Could you check a few things on this drawing? It's one solid part, dimensions in mm from its lowest x, y, z. A direction names the side the tool comes from. Round coordinates to 2 decimals unless told otherwise and drop trailing zeros. Order: outer loops, then holes, each group sorted by start corner. A loop starts at its lowest first (then second) coordinate and runs counter-clockwise, first axis right, second up.
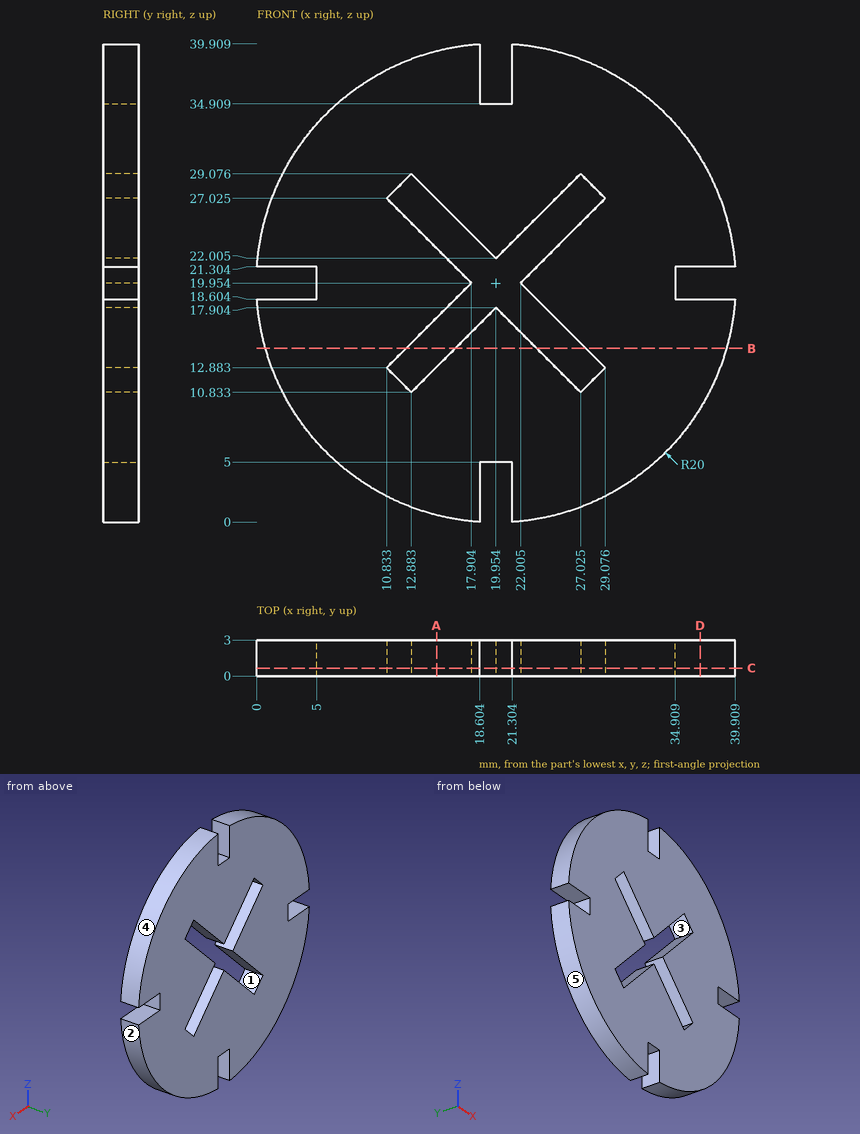
(1) I want a section at A-A, the plane x = 15. List the corners of the cut face in (y, z) for me.
(2) I'm going to push flat-ended pins straight in: pin 1 Ø1.4 at (x, y) = (19.5, 1) entering from -Z; pin 2 Ø0.9 at (y, z) = (1, 37.5) entering from -X (1 decimal); pin 3 Ø1.5 at (x, y) = (1.5, 1) entering from +Z (1 decimal). Where does each tip first touch, or does it pass through?
(3) I want a section at B-B, the plane z = 14.5. List the corners of the cut face in (x, y) for me.
(4) I want a section at D-D, the plane x = 37. List the corners of the cut face in (y, z) for me (1 decimal).
(5) If we mould it in two halves opening along X, with no side actions, what happens to the marked faces 3, 4 and 5? For each: pulls with the +X half, pulls with the -X half, needs draft (parallel to the pull), parting line crosses it, or undercut.
(6) Please list where these lines run through material, in increasing order: probe 1 along X at (y, z) = (1.6, 24); probe 2 along Z at (x, y) = (19, 1.5); probe 3 along Z at (x, y) = (2.5, 2.8) (1 decimal).
(7) On a 3-axis mill with a long thin cutter (end or side, diameter ignored), from which of +Z, -Z, +X, -X, +Y, -Y can I reach the whole of each face in a straight line? I mean the marked faces 1 and 2. Say none if no direction works.
(8) I want a section at C-C, the plane y = 0.65. List the corners of the cut face in (x, z) for me (1 decimal), plus the area to 3 significant figures.
Ans:
1. outline: (0, 0.58) - (3, 0.58) - (3, 12.95) - (0, 12.95) - close; (0, 17.05) - (3, 17.05) - (3, 22.86) - (0, 22.86) - close; (0, 26.96) - (3, 26.96) - (3, 39.33) - (0, 39.33) - close
2. pin 1: stops at z = 5
2. pin 2: stops at x = 9.6
2. pin 3: stops at z = 29.3
3. outline: (0.71, 0) - (12.45, 0) - (12.45, 3) - (0.71, 3) - close; (16.55, 0) - (23.36, 0) - (23.36, 3) - (16.55, 3) - close; (27.46, 0) - (39.2, 0) - (39.2, 3) - (27.46, 3) - close
4. outline: (0, 9.5) - (3, 9.5) - (3, 18.6) - (0, 18.6) - close; (0, 21.3) - (3, 21.3) - (3, 30.4) - (0, 30.4) - close
5. face 3: undercut
5. face 4: pulls with the +X half
5. face 5: pulls with the -X half
6. probe 1: x = 0.37 to 13.86, 17.96 to 21.95, 26.05 to 39.54
6. probe 2: z = 5 to 16.95, 22.96 to 34.91
6. probe 3: z = 10.2 to 18.6, 21.3 to 29.7
7. face 1: +Y, -Y
7. face 2: -Z, +X, +Y, -Y
8. outline: (0, 18.6) arc R20 ccw to (18.6, 0) - (18.6, 5) - (21.3, 5) - (21.3, 0) arc R20 ccw to (39.9, 18.6) - (34.9, 18.6) - (34.9, 21.3) - (39.9, 21.3) arc R20 ccw to (21.3, 39.9) - (21.3, 34.9) - (18.6, 34.9) - (18.6, 39.9) arc R20 ccw to (0, 21.3) - (5, 21.3) - (5, 18.6) - close; hole (10.8, 12.9) - (12.9, 10.8) - (20, 17.9) - (27, 10.8) - (29.1, 12.9) - (22, 20) - (29.1, 27) - (27, 29.1) - (20, 22) - (12.9, 29.1) - (10.8, 27) - (17.9, 20) - close
8. area: 1,080 mm2
